Autodesk Inventor part; units mm, degrees
ref_plane "Work Plane1" through (-6, -9, 0) normal (1, 0, 0) x (0, 1, 0)
ref_plane "XZ Plane" through (0, 0, 0) normal (0, 1, 0) x (-1, 0, 0)
ref_plane "XY Plane" through (0, 0, 0) normal (0, 0, 1) x (1, 0, 0)
sketch "Sketch1" plane through (0, 0, 0) normal (0, 0, 1) x (1, 0, 0)
  line L0 (0, 5.9) -> (0, -17.9) construction
  line L1 (-7, 0) -> (42, 0) construction
  line L2 (0, -14.5) -> (0, 2.5)
  line L3 (0, -14.5) -> (6, -14.5)
  line L4 (6, -14.5) -> (6, -3.5)
  line L5 (7, -2.5) -> (35, -2.5)
  line L6 (35, -2.5) -> (35, 2.5)
  line L7 (35, 2.5) -> (0, 2.5)
  arc A0 (7, -2.5) -> (6, -3.5) centre (7, -3.5) ccw
  point P0 (0, 0)
  point P1 (6, -2.5)
  dimension "d0" = 6
  dimension "d2" = 5
  dimension "d3" = 12
  dimension "d4" = 1
  dimension "d12" = 35
revolve "Revolution1" add sketch "Sketch1" angle 360 about axis through (0, 0, 0) along (0, -1, 0)
sketch "Sketch2" plane through (0, 2.5, 0) normal (0, -1, 0) x (1, 0, 0)
  circle A0 centre (0, 0) radius 35 construction
  circle A1 centre (0, 0) radius 7 construction
  circle A2 centre (0, 0) radius 6 construction
  line L0 (-49, 0) -> (49, 0) construction
  line L1 (0, 49) -> (0, -49) construction
  circle A3 centre (0, 0) radius 6 construction
  circle A4 centre (0, 0) radius 21.25 construction
  circle A5 centre (0, 0) radius 30 construction
  point P0 (0, 30)
  point P1 (0, 21.25)
  point P2 (-21.2132, 21.2132)
  point P3 (-15.026, 15.026)
  point P4 (-30, 0)
  point P5 (-21.25, 0)
  point P6 (-21.2132, -21.2132)
  point P7 (-15.026, -15.026)
  point P8 (0, -30)
  point P9 (0, -21.25)
  point P10 (21.2132, -21.2132)
  point P11 (15.026, -15.026)
  point P12 (30, 0)
  point P13 (21.25, 0)
  point P14 (21.2132, 21.2132)
  point P15 (15.026, 15.026)
  dimension "d6" = 42.5
  dimension "d7" = 60
  dimension "d10" = 360
hole "Hole1" at (-15.026, 2.5, 15.026) at (0, 2.5, 21.25) at (15.026, 2.5, 15.026) at (21.25, 2.5, 0) at (15.026, 2.5, -15.026) at (0, 2.5, -21.25) at (-15.026, 2.5, -15.026) at (-21.25, 2.5, 0) direction (0, -1, 0) diameter 3.4 end through all counterbore diameter 6.5 counterbore depth 3
hole "Hole2" at (0, 2.5, 30) at (-21.2132, 2.5, 21.2132) at (-30, 2.5, 0) at (-21.2132, 2.5, -21.2132) at (0, 2.5, -30) at (21.2132, 2.5, -21.2132) at (30, 2.5, 0) at (21.2132, 2.5, 21.2132) direction (0, -1, 0) diameter 3.242 end through all
ref_plane "Work Plane1" through (-6, -9, 0) normal (1, 0, 0) x (0, 1, 0)
sketch "Sketch3" plane through (-6, -9, 0) normal (1, 0, 0) x (0, 1, 0)
  line L0 (-8.9, 0) -> (14.9, 0) construction
  line L1 (-2.5, -2) -> (2.5, -2)
  line L2 (2.5, 2) -> (-2.5, 2)
  arc A0 (-2.5, 2) -> (-2.5, -2) centre (-2.5, 0) ccw
  arc A1 (2.5, -2) -> (2.5, 2) centre (2.5, 0) ccw
  line L3 (5.5, 6) -> (5.5, -6) construction
  line L4 (-5.5, 6) -> (-5.5, -6) construction
  line L5 (5.5, 6) -> (-5.5, 6) construction
  line L6 (0, 6) -> (0, -7.95) construction
  point P0 (9, 0)
  dimension "d27" = 4
  dimension "d29" = 5
extrude "Extrusion1" cut sketch "Sketch3" along normal blind 2
chamfer "Chamfer1" distance 0.5 angle 45 1 edges at (-6, -14.5, 0)
properties part number "Adapter_bearing_link"
Can you work these out from the model? Positions are in its coordinate system, mm. A direction names the side the tool comes from. Give positions to 0.01 mm unless a question says otherwise; leave off trailing zeros. Loops run counter-clockwise (first coordinate to the right, second up) from the corner with the lowest first, then second, coordinate; pieces in that order, holes last. Notation, with made-up numbers: M 88,78.5 L 142,78.5 A13 cw 142,100.5 Z; hole C 69.25,-29 d3. An arc over 180 degrees is marked long. Use CSV: the item, a comma, the result in double quotes. Start each with the question number.
1. Imagine slicing it at D-D, the plane y = -10. Write out the boundary of the cut face in (x, z), plus the area to 3 significant figures.
2. If I drill on L1, parallel to Z at x = 0, y = -1.4; L2, parallel to Y at x = -5.5, z = 19.5; L3, parallel to X at y = 0, z = 16, over which ranges is the centre line in solid material (lowest first)?
3. If we mould it in two halves opening along Z, with no side actions, what happens to faces 4 (the face through (0, -14.5, 0)), 5 (the face through (-4, -9, 0)), 6 (the face through (5.723, -8.676, -1.802))? For each: released by +Z, released by -Z, zero draft, split by the parting line, or undercut.
4. For P1, Ø5, axis at y = -1, z = -28, coming from the -X side; P2, Ø1, axis at x = -6, y = -3.5, coming from the +Z side; P3, Ø4, axis at x = 0, z = 21.25, coming from the +Y side; P4, Ø2.5, axis at x = 15.026, z = 15.026, coming from the +Y side, each with a flat end and sliding along its axis, tell me the tip position at first contact or that it passes through.
5. Imagine slicing it at A-A, the plane x = -30. Write out the boundary of the cut face in (y, z).
6. On a 3-axis mill with a long thin cutter (end or side, diameter ignored), from which of +Z, -Z, +X, -X, +Y, -Y can I reach the whole of each face in a straight line? I mean faces 1 (the face through (-5, -4.5, 0)), 2 (the face through (1.4, -0.5, -19.9)), 3 (the face through (16.06, -1.514, -16.375)). Say none if no direction works.
7. Imagine slicing it at B-B, the plane z = 0. Count the separate pieces of the cut face and the enclosed holes in it, plus the area to 3 significant figures.
Response values:
1,outline,"M -5.66,-2 A6 ccw long -5.66,2 L -4,2 L -4,-2 Z"
1,area,"106 mm^2"
2,L1,"-35 to -31.62, -28.38 to -22.95, -19.55 to 19.55, 22.95 to 28.38, 31.62 to 35"
2,L2,"-2.5 to 2.5"
2,L3,"-31.13 to -18.13, -11.93 to 11.93, 18.13 to 31.13"
3,face 4,"zero draft"
3,face 5,"undercut"
3,face 6,"split by the parting line"
4,P1,"x = -23.97"
4,P2,"z = 2.4"
4,P3,"y = -0.5"
4,P4,"through"
5,outline,"M -2.5,-18.03 L 2.5,-18.03 L 2.5,-1.62 L -2.5,-1.62 Z; M -2.5,1.62 L 2.5,1.62 L 2.5,18.03 L -2.5,18.03 Z"
6,face 1,"-X"
6,face 2,"+Y"
6,face 3,"+Y, -Y"
7,separate pieces,"5"
7,enclosed holes,"0"
7,area,"391 mm^2"
